Input: part model. Units: mm. Frame: model coordinates. Face numbers are marked on the shaded views. A direction names the side the tool comes from. Coordinates: 2 decimals unless noted, no trailing zeros. Order: outer loops, then holes, each group sorted by start corner. A loop starts at its lowest first (then second) coordinate and runs counter-clockwise, first axis right, second up. Notation, with made-up numbers: M 41.5,79.5 L 46.5,79.5 A16 cw 46.5,106.5 Z; hole C 76.5,10.25 d8. An arc over 180 degrees is marked long. Answer in a Markdown table with one row per item.
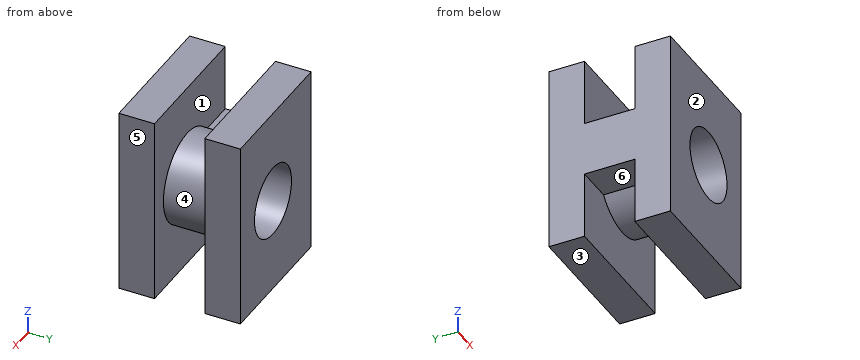
Autodesk Inventor part; units mm, degrees
ref_plane "YZ Plane" through (0, 0, 0) normal (1, 0, 0) x (0, 1, 0)
ref_plane "XZ Plane" through (0, 0, 0) normal (0, 1, 0) x (-1, 0, 0)
ref_plane "XY Plane" through (0, 0, 0) normal (0, 0, 1) x (1, 0, 0)
sketch "Sketch1" plane through (0, 0, 0) normal (0, 1, 0) x (-1, 0, 0)
  arc A0 (1.75, 1.3) -> (1.75, -1.3) centre (0, 0) ccw
  circle A1 centre (0, 0) radius 1.7
  line L0 (0, 0) -> (0, 1.3)
  line L1 (3.5, 1.3) -> (3.5, -1.3)
  line L2 (0, 1.3) -> (1.0954, 1.3)
  line L3 (1.75, 1.3) -> (3.5, 1.3)
  line L4 (3.5, -1.3) -> (1.75, -1.3)
  dimension "d1" = 3.4
  dimension "d0" = 4.36
  dimension "d2" = 1.3
  dimension "d3" = 3.5
  dimension "d4" = 2.6
extrude "Extrusion1" add sketch "Sketch1" along normal blind 2.4
sketch "Sketch2" plane through (0, 2.4, 0) normal (0, 1, 0) x (1, 0, 0)
  circle A0 centre (0, 0) radius 1.7
  line L0 (0, 0) -> (0, 4.5)
  line L1 (0, 4.5) -> (3, 4.5)
  line L2 (3, 4.5) -> (-3.5, 4.5)
  line L3 (-3.5, 4.5) -> (-3.5, -4.5)
  line L4 (-3.5, -4.5) -> (3, -4.5)
  line L5 (3, -4.5) -> (3, 4.5)
  dimension "d7" = 4.5
  dimension "d8" = 3
  dimension "d9" = 9
extrude "Extrusion2" add sketch "Sketch2" along normal blind 1.7
sketch "Sketch3" plane through (0, 0, 0) normal (0, -1, 0) x (1, 0, 0)
  line L0 (-3.5, 4.5) -> (3, 4.5)
  line L1 (3, 4.5) -> (3, -4.5)
  line L2 (-3.5, 4.5) -> (3, 4.5)
  line L3 (3, 4.5) -> (3, -4.5)
  line L4 (3, -4.5) -> (-3.5, -4.5)
  line L5 (-3.5, -4.5) -> (-3.5, 4.5)
  point P0 (0, 0)
extrude "Extrusion3" add sketch "Sketch3" along normal blind 1.7
sketch "Sketch4" plane through (0, 0, 0) normal (0, 1, 0) x (1, 0, 0)
  circle A0 centre (0, 0) radius 1.7
extrude "Extrusion4" cut sketch "Sketch4" against normal blind 1.7
properties part number "MMAE 232 CAD Assignment 2 Rubber Grommet-Nicholas Skiba"
1) Contact query for flat-ended pins moving along their axis: pin 1 (2 mm diameter, centred on y = 2, z = 1.5, fed in from +X); pin 2 (1 mm diameter, centred on x = 0, z = 0, fed in from -Y); pin 3 (0.5 mm diameter, centred on x = -2.5, y = 1, fed in from +Z). Output: stop coordinate, or through.
Resolved:
| item | result |
|---|---|
| pin 1 | stops at x = 3 |
| pin 2 | passes through |
| pin 3 | stops at z = 1.3 |
2) Cut plane A-A, the plane z = 3. Output: boundary loops of the cut face in (x, y).
Resolved:
| item | result |
|---|---|
| outline | M -3.5,-1.7 L 3,-1.7 L 3,0 L -3.5,0 Z; M -3.5,2.4 L 3,2.4 L 3,4.1 L -3.5,4.1 Z |
3) Cut plane B-B, the plane y = 3.2. Output: boundary loops of the cut face in (x, z), and give its area (3 significant figures).
Resolved:
| item | result |
|---|---|
| outline | M -3.5,-4.5 L 3,-4.5 L 3,4.5 L -3.5,4.5 Z; hole C 0,0 d3.4 |
| area | 49.4 mm2 |
4) Reachability of the marked faces 4, 5 and 6 from +Z, -Z, +X, -X, +Y, -Y: full face, straight path, thin tool, end or side. Return the list, or none.
Resolved:
| item | result |
|---|---|
| face 4 | none |
| face 5 | +Z, -Z, +X, +Y, -Y |
| face 6 | -Z, -X |
5) Material intervals for probe 1 along X at (y, z) = (2.9, 0); probe 2 along Y at (x, z) = (2.5, 0.75); probe 3 along Z at (x, y) = (0, 1.3), sorted ascending.
Resolved:
| item | result |
|---|---|
| probe 1 | x = -3.5 to -1.7, 1.7 to 3 |
| probe 2 | y = -1.7 to 0, 2.4 to 4.1 |
| probe 3 | z = -2.18 to -1.7, 1.7 to 2.18 |
6) Cut plane D-D, the plane y = 0.7. Output: boundary loops of the cut face in (x, z), and give its area (3 significant figures).
Resolved:
| item | result |
|---|---|
| outline | M -3.5,-1.3 L -1.75,-1.3 A2.18 ccw long -1.75,1.3 L -3.5,1.3 Z; hole C 0,0 d3.4 |
| area | 9.64 mm2 |
7) Mould query, pull axis Y, two halves, no side actions, for the marked faces 1, 2 and 3. Classes: +Y half, -Y half, draft (parallel to the pull), parting line (faces both ways), or undercut.
Resolved:
| item | result |
|---|---|
| face 1 | undercut |
| face 2 | -Y half |
| face 3 | draft |
